```python
from build123d import *

# Parameters (mm, degrees)
SKETCH_1_W          = 33
SKETCH_1_H          = 33
SKETCH_1_W_2        = 13
SKETCH_1_H_2        = 13
EXTRUDE_1_DEPTH     = 15
SKETCH_2_W          = 25
SKETCH_2_H          = 25
CUT_EXTRUDE_1_DEPTH = 11
FILLET_3_R          = 3
SKETCH_4_R          = 1
CUT_EXTRUDE_2_DEPTH = 43.930175867


with BuildPart() as part:
    # Эскиз1 → Бобышка-Вытянуть1 (new body)
    with BuildSketch(Plane(origin=(0, 0, 0), x_dir=(1, 0, 0), z_dir=(0, 1, 0))):
        with Locations((6.5, 6.5)):
            Rectangle(SKETCH_1_W, SKETCH_1_H)
        with Locations((6.5, 6.5)):
            Rectangle(SKETCH_1_W_2, SKETCH_1_H_2, mode=Mode.SUBTRACT)
    extrude(amount=EXTRUDE_1_DEPTH)

    # Эскиз2 → Вырез-Вытянуть1 (cut)
    with BuildSketch(Plane(origin=(0, 15, 0), x_dir=(1, 0, 0), z_dir=(0, 1, 0))):
        with Locations((6.5, 6.5)):
            Rectangle(SKETCH_2_W, SKETCH_2_H)
    extrude(amount=-CUT_EXTRUDE_1_DEPTH, mode=Mode.SUBTRACT)

    # Скругление3
    fillet_3_edges = [part.edges().sort_by_distance(p)[0] for p in [
        (6.5, 0, -23),
        (23, 0, -6.5),
        (6.5, 0, 10),
        (-10, 0, -6.5),
        (-10, 7.5, -23),
        (23, 7.5, -23),
        (23, 7.5, 10),
        (-10, 7.5, 10),
    ]]
    fillet(fillet_3_edges, radius=FILLET_3_R)

    # Эскиз4 → Вырез-Вытянуть2 (cut, through all)
    with BuildSketch(Plane.ZY.offset(10)):
        with Locations((2.75, 11)):
            Circle(SKETCH_4_R)
        with Locations((-15.75, 11)):
            Circle(SKETCH_4_R)
    extrude(amount=-CUT_EXTRUDE_2_DEPTH, mode=Mode.SUBTRACT)


solid = part.part
```
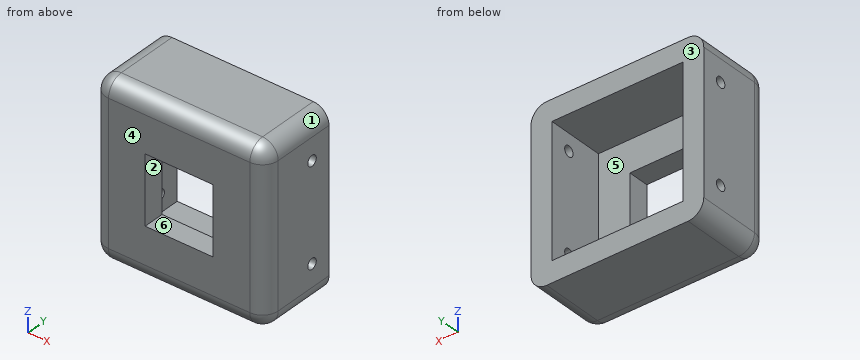
Here's how the part is built. I have some questions about the finished solid (model axes, mm). Face numbers are marked on the shaded views. A direction names the side the tool comes from. Give positions to 0.01 mm unless a question says otherwise; leave off trailing zeros. Loops run counter-clockwise (first coordinate to the right, second up) from the corner with the lowest first, then second, coordinate; pieces in that order, holes last. Notation, with made-up numbers: (88.25, 30.5) -> (128.25, 30.5) arc R28 ccw to (128.25, 65.5) -> close; hole circle Ø11 at (-40, 16.25). An arc over 180 degrees is marked (long way). Use one line per item in the form item = value. Start each with the question number.
1) For P1, Ø2, axis at x = 2.5, z = -16.5, coming from the +Y side; P2, Ø1.2, axis at y = 2, z = -5, coming from the +X side, each with a flat end and sliding along its axis, tell me the tip position at first contact or that it passes through.
2) Which directions (+Z, -Z, +X, -X, +Y, -Y) give clear straight access to the entire face, cutting with the end or side of a thin tool? Please do the marked faces 4, 5 and 6.
3) Imagine slicing it at C-C (z = -6). Please give me the cut outline in (x, y), then the cut area to 3 significant figures.
4) Thinking about a two-plate mould opening in Z: for the marked faces 1, 2 and 3, which applies, +Z half, -Z half, draft (parallel to the pull), parting line (faces both ways), or undercut?
5) Imagine slicing it at B-B (x = 1.5). Please give me the cut outline in (y, z).
6) Imagine slicing it at A-A (y = 11). Please give me the cut outline in (x, z), then the cut area to 3 significant figures.
7) Please list where these lines run through material, in increasing order: line 1 along X through (y, z) = (13, -10); line 2 along Z through (x, y) = (18.5, 12.75); line 3 along Y through (x, z) = (20.2, -15.75).
8) Imagine slicing it at D-D (z = 2.75). Please give me the cut outline in (x, y).
Check values:
q1.P1 = 4
q1.P2 = 22.97
q2.face_4 = +Z, -Z, +X, -X, -Y
q2.face_5 = +Y
q2.face_6 = +Y, -Y
q3.outline = (-10, 3) arc R3 ccw to (-7, 0) -> (0, 0) -> (0, 4) -> (-6, 4) -> (-6, 15) -> (-10, 15) -> close; (13, 0) -> (20, 0) arc R3 ccw to (23, 3) -> (23, 15) -> (19, 15) -> (19, 4) -> (13, 4) -> close
q3.area = 164 mm^2
q4.face_1 = +Z half
q4.face_2 = undercut
q4.face_3 = draft
q5.outline = (0, -20) arc R3 ccw to (3, -23) -> (15, -23) -> (15, -19) -> (4, -19) -> (4, -13) -> (0, -13) -> close; (0, 0) -> (4, 0) -> (4, 6) -> (15, 6) -> (15, 10) -> (3, 10) arc R3 ccw to (0, 7) -> close
q6.outline = (-10, -20) arc R3 ccw to (-7, -23) -> (20, -23) arc R3 ccw to (23, -20) -> (23, -16.75) -> (19, -16.75) -> (19, -19) -> (-6, -19) -> (-6, -16.75) -> (-10, -16.75) -> close; (-10, -14.75) -> (-6, -14.75) -> (-6, 1.75) -> (-10, 1.75) -> close; (-10, 3.75) -> (-6, 3.75) -> (-6, 6) -> (19, 6) -> (19, 3.75) -> (23, 3.75) -> (23, 7) arc R3 ccw to (20, 10) -> (-7, 10) arc R3 ccw to (-10, 7) -> close; (19, -14.75) -> (23, -14.75) -> (23, 1.75) -> (19, 1.75) -> close
q6.area = 424 mm^2
q7.line_1 = -10 to -6, 19 to 23
q7.line_2 = -23 to -19, 6 to 10
q7.line_3 = 0.01 to 10, 12 to 15
q8.outline = (-10, 3) arc R3 ccw to (-7, 0) -> (20, 0) arc R3 ccw to (23, 3) -> (23, 10) -> (19, 10) -> (19, 4) -> (-6, 4) -> (-6, 10) -> (-10, 10) -> close; (-10, 12) -> (-6, 12) -> (-6, 15) -> (-10, 15) -> close; (19, 12) -> (23, 12) -> (23, 15) -> (19, 15) -> close
